For this review, take the finished solid that the model builds, in its own axes (mm). A direction names the side the tool comes from. Round coordinates to 2 decimals unless told otherwise and drop trailing zeros. Order: outer loops, then holes, each group sorted by start corner. A loop starts at its lowest first (then second) coordinate and runs counter-clockwise, first axis right, second up. Notation, with made-up numbers: M 9,-24.5 L 41,-24.5 A21 ccw 41,-18.5 Z; hole C 23,33.25 d4. An arc over 180 degrees is marked long. Answer in a Markdown table with one row per item. Add a question column.
```python
from build123d import *

# Parameters (mm, degrees)
M3X0_5_TAPPED_HOLE1_D     = 2.5
M3X0_5_TAPPED_HOLE1_DEPTH = 7.5
M3X0_5_TAPPED_HOLE1_TIP   = 0.751075774
SKETCH5_R                 = 30.5
BOSS_EXTRUDE1_DEPTH       = 3


with BuildPart() as part:
    # Sketch1 → Revolve1 (revolve)
    with BuildSketch(Plane.XY, mode=Mode.PRIVATE) as revolve1_sk:
        Polygon((-6.6, 0), (6.6, 0), (6.6, 26.5), (1, 26.5), (-0.4, 31.5), (-6.6, 31.5), align=None)
    revolve(revolve1_sk.sketch.rotate(Axis((-6.6, 0, 0), (1, 0, 0)), 180), axis=Axis((-6.6, 0, 0), (1, 0, 0)))

    # M3x0.5 Tapped Hole1
    with Locations(Plane(origin=(6.6, 0, 0), x_dir=(0, 0, -1), z_dir=(1, 0, 0))):
        with Locations((-10.606601718, 10.606601718), (-10.606601718, -10.606601718), (10.606601718, -10.606601718), (10.606601718, 10.606601718)):
            Hole(M3X0_5_TAPPED_HOLE1_D / 2, depth=M3X0_5_TAPPED_HOLE1_DEPTH)
            with Locations((0, 0, -(M3X0_5_TAPPED_HOLE1_DEPTH + M3X0_5_TAPPED_HOLE1_TIP / 2))):  # 118° drill point
                Cone(0, M3X0_5_TAPPED_HOLE1_D / 2, M3X0_5_TAPPED_HOLE1_TIP, mode=Mode.SUBTRACT)

    # Sketch5 → Boss-Extrude1 (add)
    with BuildSketch(Plane.ZY.offset(6.6)):
        with Locations(Location((0, 0, 0), (0, 0, 270))):
            Circle(SKETCH5_R)
    extrude(amount=BOSS_EXTRUDE1_DEPTH)


solid = part.part
```
1. Consider section D-D on x = 4. Write out the cut boundary in (y, z), plus the area to 3 significant figures.
2. Consider section A-A on z = 0. Write out the cut boundary in (x, y).
3. For faces 4 (the cylindrical face through (2.797, -11.827, 10.336)), 5 (the cylindrical face through (-3.543, 4.101, -31.232)), 6 (the cylindrical face through (-8.079, 6.612, -29.775)), list the 3-axis set-ups (+Z, -Z, +X, -X, +Y, -Y) from which the entire face can be reached by the end or side of a thin tool; tool diameter is ignored.
4. The part is to be moulded in two halves that separate along Z. For faces 1 (the flat face through (6.6, 0, 0)), 2 (the conical face through (0.91, 5.81, 26.18)), 3 (the conical face through (-1.52, 10.75, 10.77)), say which applies: pulls with the +Z half, pulls with the -Z half, needs draft (parallel to the pull), parting line crosses it, or undercut.
5. To check wall thickness, follow probe 1 along Z at (x, y) = (4.5, 11.5); probe 2 along Z at (x, y) = (-3, -15); probe 3 along Y at (x, z) = (5.5, 3). State the ranges of each line that lie inside material, in increasing order. Write a range as [from, to].
6. Consider section C-C on x = -8.5. Write out the cut boundary in (y, z), plus the area to 3 significant figures.
7. Clearance check with flat-ended pins moving along their axes: pin 1 Ø8 at (x, y) = (-6, 13.5) entering from +Z; pin 2 Ø2 at (y, z) = (10.61, -10.61) entering from +X; pin 3 Ø2 at (x, y) = (-2.5, -15.5) entering from -Z. State where each tip first meets the part, or that it passes through.
Solved:
| question | item | result |
|---|---|---|
| 1 | outline | C 0,0 d53; hole C -10.61,-10.61 d2.5; hole C -10.61,10.61 d2.5; hole C 10.61,-10.61 d2.5; hole C 10.61,10.61 d2.5 |
| 1 | area | 2,190 mm^2 |
| 2 | outline | M -9.6,-30.5 L -6.6,-30.5 L -6.6,-31.5 L -0.4,-31.5 L 1,-26.5 L 6.6,-26.5 L 6.6,26.5 L 1,26.5 L -0.4,31.5 L -6.6,31.5 L -6.6,30.5 L -9.6,30.5 Z |
| 3 | face 4 | +X |
| 3 | face 5 | +X, -X |
| 3 | face 6 | -X |
| 4 | face 1 | needs draft |
| 4 | face 2 | parting line crosses it |
| 4 | face 3 | undercut |
| 5 | probe 1 | z = [-23.87, -11.48], [-9.73, 9.73], [11.48, 23.87] |
| 5 | probe 2 | z = [-27.7, 27.7] |
| 5 | probe 3 | y = [-26.33, 26.33] |
| 6 | outline | C 0,0 d61 |
| 6 | area | 2,920 mm^2 |
| 7 | pin 1 | stops at z = 30.03 |
| 7 | pin 2 | stops at x = -1.05 |
| 7 | pin 3 | stops at z = -27.96 |
